Geometry: see drawing. Coordinates: mm, zero at the bounding-box minimum. Coordinates: 2 decimals unless noted, no trailing zeros. Loops run counter-clockwise (first coordinate to the right, second up) from the corner with the lowest first, then second, coordinate; pieces in that order, holes last. Notation, with made-up numbers: (78.5, 44) -> (111.5, 44) arc R21 ccw to (111.5, 67) -> close; hole circle Ø7 at (33, -12). An arc over 180 degrees is marked (long way). Answer as a JSON object with one key per item and string values.
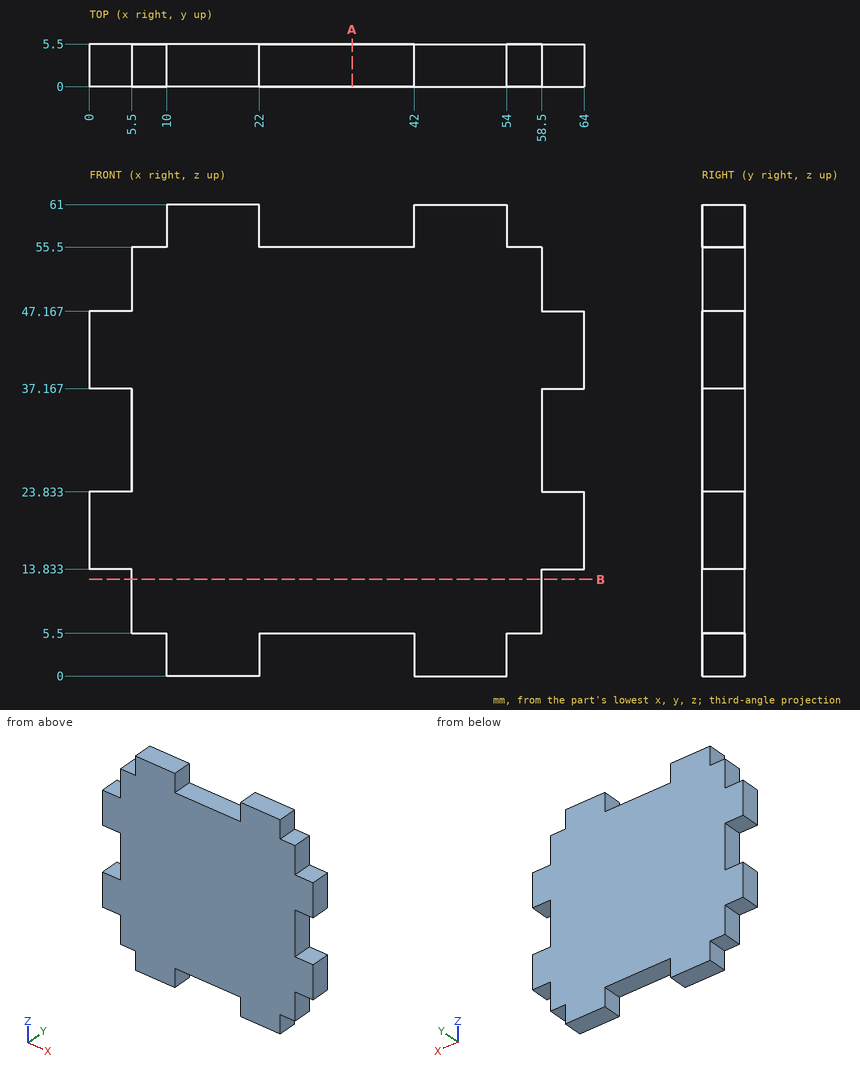
1. Section query A-A (x = 34). Return loops of the section in (y, z).
Reply:
{"outline": "(0, 5.5) -> (5.5, 5.5) -> (5.5, 55.5) -> (0, 55.5) -> close"}
2. Pin query (flat end, axial travel): P1, Ø1.6, axis at x = 60, y = 2, coming from the +Z side; P2, Ø3, axis at x = 2.5, y = 3.5, coming from the -Z side; P3, Ø1.6, axis at y = 1.5, z = 58.5, coming from the -X side. Return the tip coordinate at first contact, or that it passes through.
Reply:
{"P1": "stops at z = 47.17", "P2": "stops at z = 13.83", "P3": "stops at x = 10"}
3. Section query B-B (z = 12.5). Return loops of the section in (x, y).
Reply:
{"outline": "(5.5, 0) -> (58.5, 0) -> (58.5, 5.5) -> (5.5, 5.5) -> close"}
4. Line query: line 1 along X through (y, z) = (5, 58); line 2 along Z through (x, y) = (23, 2.65); line 3 along X through (y, z) = (4.65, 54). Output: solid intervals per line, ascending.
Reply:
{"line 1": "x = 10 to 22, 42 to 54", "line 2": "z = 5.5 to 55.5", "line 3": "x = 5.5 to 58.5"}
